Model file for the job. Use its own axes, mm. Coordinates: 2 decimals unless noted, no trailing zeros. Order: outer loops, then holes, each group sorted by start corner. A loop starts at its lowest first (then second) coordinate and runs counter-clockwise, first axis right, second up. Notation, with made-up numbers: (29.25, 66.5) -> (78.25, 66.5) arc R17 ccw to (78.25, 85.5) -> close; hole circle Ø3 at (-10, -36.75). An arc over 180 degrees is marked (long way). Use CSV: the item, a comma, the result in double quotes. Start each with the question number.
(1) Cut at D-D on y = 146. Write the cut outline in (x, z), plus the area to 3 significant figures.
(2) Cut at B-B on y = 190.5. Write the cut outline in (x, z), plus the area to 3 significant figures.
(3) Pin check, flat tips, straight feed: pin 1 Ø6 at (y, z) = (115.5, 5) entering from -X; pin 2 Ø6 at (y, z) = (190.5, 0) entering from +X (3 decimals); pin 3 Ø1.5 at (x, y) = (-2.5, 135) entering from +Z; pin 4 Ø4.5 at (y, z) = (194.5, -1) entering from -X. Stop position of each tip, or through.
(4) Cut at A-A on z = 0. Write the cut outline in (x, y).
(5) Probe L1, parallel to Y at x = 3, z = 0; L2, parallel to X at y = 97.5, z = -9; L3, parallel to Y at x = -3.75, z = -2. List the from-to ranges inside material, lowest first.
(6) Cut at C-C on x = -6.75. Write the cut outline in (y, z), plus the area to 3 significant figures.
```python
from build123d import *

# Parameters (mm, degrees)
SKETCH_1_R          = 10
EXTRUDE_1_DEPTH     = 200
CUT_EXTRUDE_START   = -19
CUT_EXTRUDE_1_DEPTH = 19
SKETCH_3_R          = 3.25
CUT_EXTRUDE_4_DEPTH = 202.149198358


with BuildPart() as part:
    # 草图1 → 凸台-拉伸1 (new body)
    with BuildSketch(Plane(origin=(0, 0, 0), x_dir=(1, 0, 0), z_dir=(0, 1, 0))):
        with Locations(Location((0, 0, 0), (0, 0, 270))):
            Circle(SKETCH_1_R)
    extrude(amount=EXTRUDE_1_DEPTH)

    # 草图2 → 切除-拉伸1 (cut)
    with BuildSketch(Plane(origin=(0, 200, 0), x_dir=(1, 0, 0), z_dir=(0, 1, 0)).offset(CUT_EXTRUDE_START)):
        with BuildLine():
            Line((-9, -4.358898944), (-9, 4.358898944))
            ThreePointArc((-9, 4.358898944), (-10, 0), (-9, -4.358898944))
        make_face()
        with BuildLine():
            ThreePointArc((10, 0), (9.746794345, 2.236067977), (9, 4.358898944))
            Line((9, 4.358898944), (9, -4.358898944))
            ThreePointArc((9, -4.358898944), (9.746794345, -2.236067977), (10, 0))
        make_face()
    extrude(amount=CUT_EXTRUDE_1_DEPTH, mode=Mode.SUBTRACT)

    # 草图3 → 切除-拉伸4 (cut, through all)
    with BuildSketch(Plane.ZY.offset(9)):
        with Locations((0, 190.5)):
            Circle(SKETCH_3_R)
    extrude(amount=-CUT_EXTRUDE_4_DEPTH, mode=Mode.SUBTRACT)


solid = part.part
```
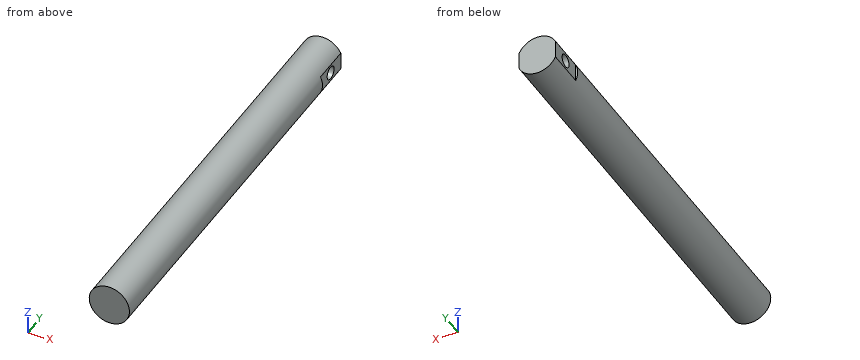
Outcome:
1,outline,"circle Ø20 at (0, 0)"
1,area,"314 mm2"
2,outline,"(-9, -4.36) arc R10 ccw to (9, -4.36) -> (9, -3.25) -> (-9, -3.25) -> close; (-9, 3.25) -> (9, 3.25) -> (9, 4.36) arc R10 ccw to (-9, 4.36) -> close"
2,area,"185 mm2"
3,pin 1,"x = -9.8"
3,pin 2,"through"
3,pin 3,"z = 9.85"
3,pin 4,"x = -9"
4,outline,"(-10, 0) -> (10, 0) -> (10, 181) -> (9, 181) -> (9, 187.25) -> (-9, 187.25) -> (-9, 181) -> (-10, 181) -> close; (-9, 193.75) -> (9, 193.75) -> (9, 200) -> (-9, 200) -> close"
5,L1,"0 to 187.25, 193.75 to 200"
5,L2,"-4.36 to 4.36"
5,L3,"0 to 187.94, 193.06 to 200"
6,outline,"(0, -7.38) -> (200, -7.38) -> (200, 7.38) -> (0, 7.38) -> close; hole circle Ø6.5 at (190.5, 0)"
6,area,"2,920 mm2"
